```python
from build123d import *

# Parameters (mm, degrees)
F0_R     = 0.5
F0_R_2   = 1.65
F1_DEPTH = 33.5


with BuildPart() as f1:
    # F0 (on Top) → F1 (new body)
    with BuildSketch(Plane.XY):
        with BuildLine():
            Line((-12.55, 42.4), (-29.15, 42.4))
            Line((-29.15, 42.4), (-29.15, 0.5))
            ThreePointArc((-29.15, 0.5), (-28.7964466094, 0.3535533906), (-28.65, 0))
            ThreePointArc((-28.65, 0), (-28.7964466094, -0.3535533906), (-29.15, -0.5))
            Line((-29.15, -0.5), (-29.15, -42.4))
            Line((-29.15, -42.4), (-0.5, -42.4))
            ThreePointArc((-0.5, -42.4), (0, -41.9), (0.5, -42.4))
            Line((0.5, -42.4), (20.9529261778, -42.4))
            Line((20.9529261778, -42.4), (20.9529261778, -40.0974052754))
            ThreePointArc((20.9529261778, -40.0974052754), (22.75, -38.4), (24.5470738222, -40.0974052754))
            Line((24.5470738222, -40.0974052754), (24.5470738222, -42.4))
            Line((24.5470738222, -42.4), (29.15, -42.4))
            Line((29.15, -42.4), (29.15, -0.5))
            ThreePointArc((29.15, -0.5), (28.65, 0), (29.15, 0.5))
            Line((29.15, 0.5), (29.15, 42.4))
            Line((29.15, 42.4), (20.65, 42.4))
            Line((20.65, 42.4), (20.65, 32.9))
            Line((20.65, 32.9), (-12.55, 32.9))
            Line((-12.55, 32.9), (-12.55, 42.2510281205))
            Line((-12.55, 42.2510281205), (-12.55, 42.4))
        make_face()
        with Locations((-24.15, -37.4)):
            Circle(F0_R, mode=Mode.SUBTRACT)
        with Locations((-24.5, 38.35)):
            Circle(F0_R_2, mode=Mode.SUBTRACT)
        with Locations((24.9, 37.65)):
            Circle(F0_R, mode=Mode.SUBTRACT)
        with BuildLine():
            ThreePointArc((-28.65, 0), (-28.7964466094, 0.3535533906), (-29.15, 0.5))
            Line((-29.15, 0.5), (-29.15, -0.5))
            ThreePointArc((-29.15, -0.5), (-28.7964466094, -0.3535533906), (-28.65, 0))
        make_face()
        with BuildLine():
            Line((-29.15, -0.5), (-29.15, 0.5))
            ThreePointArc((-29.15, 0.5), (-29.65, 0), (-29.15, -0.5))
        make_face()
        with BuildLine():
            ThreePointArc((0.5, -42.4), (0, -41.9), (-0.5, -42.4))
            Line((-0.5, -42.4), (0.5, -42.4))
        make_face()
        with BuildLine():
            Line((0.5, -42.4), (-0.5, -42.4))
            ThreePointArc((-0.5, -42.4), (0, -42.9), (0.5, -42.4))
        make_face()
        with BuildLine():
            ThreePointArc((29.65, 0), (29.5035533906, 0.3535533906), (29.15, 0.5))
            Line((29.15, 0.5), (29.15, -0.5))
            ThreePointArc((29.15, -0.5), (29.5035533906, -0.3535533906), (29.65, 0))
        make_face()
        with BuildLine():
            Line((29.15, -0.5), (29.15, 0.5))
            ThreePointArc((29.15, 0.5), (28.65, 0), (29.15, -0.5))
        make_face()
    extrude(amount=F1_DEPTH)


solid = f1.part
```
Input: part model. Units: mm. Frame: model coordinates. A direction names the side the tool comes from. Round coordinates to 2 decimals unless told otherwise and drop trailing zeros. Write each loop counter-clockwise with the first axis right and the second up, starting at its lowest first coordinate (ties: lowest second). Pieces come first, ordered by that corner, then holes. Notation, with made-up numbers: (7.25, 5.25) - (37.25, 5.25) arc R17 cw to (37.25, 9.25) - close; hole circle Ø1 at (84.5, -9). An arc over 180 degrees is marked (long way). Write item = value, one per line.
(1) Material intervals for probe 1 along Y at (x, z) = (24.9, 9.5); probe 2 along X at (y, z) = (-28, 11); probe 3 along Y at (x, z) = (14.5, 25), sorted ascending.
Geometry check:
probe_1 = -42.4 to 37.15, 38.15 to 42.4
probe_2 = -29.15 to 29.15
probe_3 = -42.4 to 32.9
(2) Pull-direction query (X, two-part tool) for faces 1 (the flat face through (29.15, 21, 17)), 2 (the flat face through (25, 42.4, 17)), 3 (the cylindrical face through (-25.716, 39.465, 16.516)); classes: +X half, -X half, draft (parallel to the pull), parting line (faces both ways), or undercut.
Geometry check:
face_1 = +X half
face_2 = draft
face_3 = undercut
(3) Access query for faces 4 (the flat face through (20.65, 38, 17)), 5 (the flat face through (-15, -42.4, 17)), 6 (the flat face through (24.547, -41, 17)). Directions: +Z, -Z, +X, -X, +Y, -Y. A direction counts if a zero-diameter tool reaches every point of the face in a straight line with its end or side. Return the directions, or none.
Geometry check:
face_4 = +Z, -Z, +Y
face_5 = +Z, -Z, -X, -Y
face_6 = +Z, -Z, -Y
(4) Section query A-A on z = 16.5. Output: boundary loops of the cut face in (x, y).
Geometry check:
outline = (-29.15, -42.4) - (-0.5, -42.4) arc R0.5 ccw to (0.5, -42.4) - (20.95, -42.4) - (20.95, -40.1) arc R1.8 cw to (24.55, -40.1) - (24.55, -42.4) - (29.15, -42.4) - (29.15, -0.5) arc R0.5 ccw to (29.15, 0.5) - (29.15, 42.4) - (20.65, 42.4) - (20.65, 32.9) - (-12.55, 32.9) - (-12.55, 42.4) - (-29.15, 42.4) - (-29.15, 0.5) arc R0.5 ccw to (-29.15, -0.5) - close; hole circle Ø3.3 at (-24.5, 38.35); hole circle Ø1 at (-24.15, -37.4); hole circle Ø1 at (24.9, 37.65)
(5) Section query C-C on x = 11. Output: boundary loops of the cut face in (y, z), then the cut area to 3 significant figures.
Geometry check:
outline = (-42.4, 0) - (32.9, 0) - (32.9, 33.5) - (-42.4, 33.5) - close
area = 2,520 mm^2
(6) Section query B-B on y = 8. Output: boundary loops of the cut face in (x, z), then the cut area to 3 significant figures.
Geometry check:
outline = (-29.15, 0) - (29.15, 0) - (29.15, 33.5) - (-29.15, 33.5) - close
area = 1,950 mm^2
(7) Contact query for flat-ended pins moving along their axis: pin 1 Ø3 at (x, z) = (16.5, 10.5) entering from -Y; pin 2 Ø1.5 at (y, z) = (33.5, 20) entering from +X; pin 3 Ø17 at (y, z) = (-29.5, 23) entering from -X; pin 4 Ø3 at (x, y) = (-24.5, 38.35) entering from -Z. Output: stop coordinate, or through.
Geometry check:
pin_1 = -42.4
pin_2 = 29.15
pin_3 = -29.15
pin_4 = through
